For this review, take the finished solid that the model builds, in its own axes (mm). A direction names the side the tool comes from. Give positions to 0.01 mm unless a question says otherwise; leave off trailing zeros. Order: outer loops, then holes, each group sorted by start corner. A loop starts at its lowest first (then second) coordinate and runs counter-clockwise, first axis right, second up.
Item 1: Consider section B-B (y = 9). Give the boundary of the cut face in (x, z).
Item 2: Consider section C-C (x = -51). Give the boundary of the cut face in (y, z).
Item 3: For probe 1 along Y at (x, z) = (-65, 4); probe 2 along X at (y, z) = (9, 16); probe 3 along X at (y, z) = (19, 16), list the stretches that pass through material, from the lowest coordinate up.
Item 4: Machinability: for faces 1 (the flat face through (-84, 11.418, 13)), 2 (the flat face through (-137.403, 6, 13)), 3 (the flat face through (14.997, 6, 13)), which of the approach directions +Z, -Z, +X, -X, +Y, -Y give a long, thin tool a straight path to every point of the face, cutting with its end or side? Answer none if there is none.
Item 5: Consider section A-A (z = 19.25). Give the boundary of the cut face in (x, y), plus the area to 3 significant figures.
Item 6: For P1, Ø12, axis at y = 30.5, z = 16, coming from the +X side; P2, Ø12.5, axis at y = 7, z = 17, coming from the +X side; P3, Ø3, axis at y = 12.5, z = 10, coming from the +X side, all flat-tipped, find the tip position at first contact; note any pin that passes through.
```python
from build123d import *

# Parameters (mm, degrees)
F1_DEPTH  = 25.4
F1_FACE_W = 11.417828
F1_FACE_H = 25.4
F2_DEPTH  = 152.4


with BuildPart() as f1:
    # F0 (on Top) → F1 (new body)
    with BuildSketch(Plane.XY):
        Polygon((-64.757831, 0), (14.996547, 0), (14.996547, 11.417828), (-32.038085, 11.417828), (-64.757831, 11.417828), align=None)
        Polygon((-32.038085, 11.417828), (14.996547, 11.417828), (33.608254, 36.400016), (15.166967, 43.285497), align=None)
    extrude(amount=F1_DEPTH)

    # F1_face (on face) → F2 (join)
    with BuildSketch(Plane(origin=(14.996547, 5.708914, 12.7), x_dir=(0, 1, 0), z_dir=(1, 0, 0))):
        Rectangle(F1_FACE_W, F1_FACE_H)
    extrude(amount=-F2_DEPTH)


solid = f1.part
```
Resolved:
1. outline: (-137.4, 0) - (15, 0) - (15, 25.4) - (-137.4, 25.4) - close
2. outline: (0, 0) - (11.42, 0) - (11.42, 25.4) - (0, 25.4) - close
3. probe 1: y = 0 to 11.42
3. probe 2: x = -137.4 to 15
3. probe 3: x = -20.81 to 20.65
4. face 1: +Z, -Z, -X, +Y
4. face 2: +Z, -Z, -X, +Y, -Y
4. face 3: +Z, -Z, +X, -Y
5. outline: (-137.4, 0) - (15, 0) - (15, 11.42) - (33.61, 36.4) - (15.17, 43.29) - (-32.04, 11.42) - (-137.4, 11.42) - close
5. area: 2,780 mm2
6. P1: stops at x = 33.61
6. P2: stops at x = 16.36
6. P3: stops at x = 16.92
